Model file for the job. Use its own axes, mm. A direction names the side the tool comes from. Round coordinates to 2 decimals unless told otherwise and drop trailing zeros. Write each loop counter-clockwise with the first axis right and the second up, starting at its lowest first coordinate (ties: lowest second). Pieces come first, ordered by that corner, then holes. Notation, with made-up numbers: (57, 20.25) - (68, 20.25) arc R29 ccw to (68, 41.25) - close; hole circle Ø4 at (17, -2.75). An arc over 180 degrees is marked (long way). One line per item, written item: value.
from build123d import *

# Parameters (mm, degrees)
F0_R     = 11
F1_DEPTH = 20
F2_DEPTH = 10
F3_DEPTH = 25


with BuildPart() as f1:
    # F0 (on Top) → F1 (new body, symmetric)
    with BuildSketch(Plane.XY):
        with BuildLine():
            ThreePointArc((-21.817424, -10), (5.117705, -23.448008), (24, 0))
            ThreePointArc((24, 0), (5.117705, 23.448008), (-21.817424, 10))
            ThreePointArc((-21.817424, 10), (-24, 0), (-21.817424, -10))
        make_face()
        Circle(F0_R, mode=Mode.SUBTRACT)
    extrude(amount=F1_DEPTH, both=True)

    # F0 (on Top) → F2 (join, symmetric)
    with BuildSketch(Plane.XY):
        with BuildLine():
            ThreePointArc((-21.817424, -10), (-24, 0), (-21.817424, 10))
            Line((-21.817424, 10), (-124, 10))
            Line((-124, 10), (-124, 0))
            Line((-124, 0), (-124, -10))
            Line((-124, -10), (-21.817424, -10))
        make_face()
    extrude(amount=F2_DEPTH, both=True)

    # F0 (on Top) → F3 (cut)
    with BuildSketch(Plane.XY):
        Circle(F0_R)
    extrude(amount=F3_DEPTH, mode=Mode.SUBTRACT)


solid = f1.part
1. Band-saw the part on B-B on z = 1. Write the cut outline in (x, y).
Report:
outline: (-124, -10) - (-21.82, -10) arc R24 ccw (long way) to (-21.82, 10) - (-124, 10) - close; hole circle Ø22 at (0, 0)
2. Band-saw the part on A-A on x = 0. Write the cut outline in (y, z).
Report:
outline: (-24, -20) - (-11, -20) - (-11, 20) - (-24, 20) - close; (11, -20) - (24, -20) - (24, 20) - (11, 20) - close
3. Drop flat-ended pins along their axis: pin 1 (3 mm diameter, centred on y = 16, z = -9.5, fed in from -X); pin 2 (6 mm diameter, centred on y = 13, z = -9, fed in from +X); pin 3 (12 mm diameter, centred on x = -89, z = -5.5, fed in from +Y); pin 4 (17.5 mm diameter, centred on x = 0, y = 0, fed in from +Z). Give the stop position or say it passes through.
Report:
pin 1: x = -19.12
pin 2: x = 21.82
pin 3: y = 10
pin 4: through
4. Band-saw the part on C-C on y = -16. Write the cut outline in (x, z), plus the area to 3 significant figures.
Report:
outline: (-17.89, -20) - (17.89, -20) - (17.89, 20) - (-17.89, 20) - close
area: 1,430 mm²
5. Band-saw the part on D-D on x = -72. Write the cut outline in (y, z).
Report:
outline: (-10, -10) - (10, -10) - (10, 10) - (-10, 10) - close
6. Wall check: probe 1 along Y at (x, z) = (0, -3); probe 2 along Y at (x, z) = (-23.5, -1). Give the ranges that are in metal, low to high. Write a range as [from, to].
Report:
probe 1: [-24, -11], [11, 24]
probe 2: [-10, 10]
7. Tool access for faces 1 (the face through (5, -10, -20)), 2 (the face through (-72, 10, 0)), 3 (the face through (-74, -10, 0)): list every direction of +Z, -Z, +X, -X, +Y, -Y with a clear straight run to the whole face (end or side of a thin tool).
Report:
face 1: -Z, +X, -X, +Y, -Y
face 2: +Z, -Z, -X, +Y
face 3: +Z, -Z, -X, -Y
